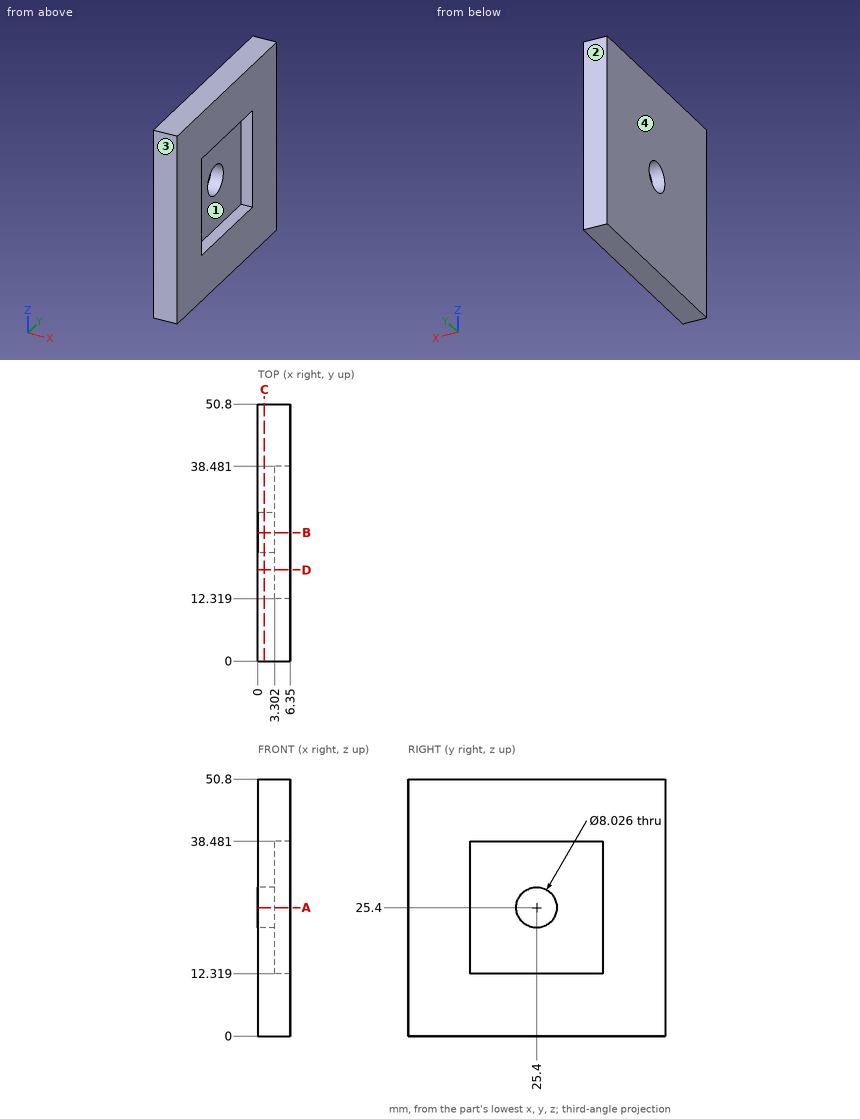
Job drawing, mm, ordinate dimensions from the low corner. One solid piece. Round coordinates to 2 decimals unless told otherwise and drop trailing zeros. Loops run counter-clockwise (first coordinate to the right, second up) from the corner with the lowest first, then second, coordinate; pieces in that order, holes last. Notation, with made-up numbers: (42.25, -18.5) -> (99.25, -18.5) arc R37 ccw to (99.25, 18.5) -> close; hole circle Ø4 at (62, 85). An arc over 180 degrees is marked (long way). One line per item, written item: value. Start each with the question number.
Q1. Cut at C-C on x = 1.25. List the corners of the cut face in (y, z), plus the area to 3 significant figures.
Q2. Probe line 1 along Z through (x, y) = (1.85, 25.4); line 2 along Y through (x, z) = (5.75, 14). List the from-to ranges inside material, lowest first.
Q3. Cut at D-D on y = 18. List the corners of the cut face in (x, z), plus the area to 3 significant figures.
Q4. Cut at A-A on z = 25.4. List the corners of the cut face in (x, y).
Q5. Two-plate mould, pull along Y, no slides. Class the marked faces 1, 2, 3 and 4: released by +Y, released by -Y, zero draft, split by the parting line, or undercut.
Q6. Drop flat-ended pins along their axis: pin 1 Ø8 at (y, z) = (28.5, 30.5) entering from +X; pin 2 Ø5 at (y, z) = (25.4, 25.4) entering from +X. Give the stop position or say it passes through.
Computed:
1. outline: (0, 0) -> (50.8, 0) -> (50.8, 50.8) -> (0, 50.8) -> close; hole circle Ø8.03 at (25.4, 25.4)
1. area: 2,530 mm²
2. line 1: 0 to 21.39, 29.41 to 50.8
2. line 2: 0 to 12.32, 38.48 to 50.8
3. outline: (0, 0) -> (6.35, 0) -> (6.35, 12.32) -> (3.3, 12.32) -> (3.3, 38.48) -> (6.35, 38.48) -> (6.35, 50.8) -> (0, 50.8) -> close
3. area: 243 mm²
4. outline: (0, 0) -> (6.35, 0) -> (6.35, 12.32) -> (3.3, 12.32) -> (3.3, 21.39) -> (0, 21.39) -> close; (0, 29.41) -> (3.3, 29.41) -> (3.3, 38.48) -> (6.35, 38.48) -> (6.35, 50.8) -> (0, 50.8) -> close
5. face 1: undercut
5. face 2: released by +Y
5. face 3: released by -Y
5. face 4: zero draft
6. pin 1: x = 3.3
6. pin 2: through
